Could you check a few things on this model? Use its own coordinates, in mm. A direction names the side the tool comes from. Round coordinates to 2 decimals unless told otherwise and drop trailing zeros. Loops run counter-clockwise (first coordinate to the right, second up) from the corner with the lowest first, then second, coordinate; pieces in that order, holes last. Notation, with made-up numbers: (60, 32.25) - (112, 32.25) arc R20 cw to (112, 53.25) - close; hole circle Ø4 at (-19, -15). An arc over 180 degrees is marked (long way). Use one line per item in the form item = value.
Autodesk Inventor part; units mm, degrees
ref_plane "YZ Plane" through (0, 0, 0) normal (1, 0, 0) x (0, 1, 0)
ref_plane "XZ Plane" through (0, 0, 0) normal (0, 1, 0) x (-1, 0, 0)
ref_plane "XY Plane" through (0, 0, 0) normal (0, 0, 1) x (1, 0, 0)
sketch "スケッチ1" plane through (0, 0, 0) normal (0, 0, 1) x (1, 0, 0)
  line L0 (-32.2352, 43.3932) -> (10.6011, 47.1409) construction
  line L1 (10.6011, 47.1409) -> (13.3901, 15.2627) construction
  line L2 (13.3901, 15.2627) -> (-29.4462, 11.515) construction
  line L3 (-29.4462, 11.515) -> (-32.2352, 43.3932) construction
  line L4 (-32.2352, 43.3932) -> (13.3901, 15.2627) construction
  line L5 (10.6011, 47.1409) -> (-29.4462, 11.515) construction
  line L6 (-30.8407, 27.4541) -> (11.9956, 31.2018) construction
  line L7 (7.8305, 44.389) -> (-19.0668, 42.0358) construction
  line L8 (-19.0668, 42.0358) -> (-16.7136, 15.1385) construction
  line L9 (-16.7136, 15.1385) -> (10.1837, 17.4917) construction
  line L10 (10.1837, 17.4917) -> (7.8305, 44.389) construction
  line L11 (7.8305, 44.389) -> (-16.7136, 15.1385) construction
  line L12 (-19.0668, 42.0358) -> (10.1837, 17.4917) construction
  circle A0 centre (-18.8864, 28.5) radius 10.5 construction
  circle A1 centre (-19.0668, 42.0358) radius 1.35
  line L13 (-5.6182, 43.2124) -> (-3.265, 16.3151) construction
  circle A2 centre (7.8305, 44.389) radius 1.35
  circle A3 centre (-16.7136, 15.1385) radius 1.35
  circle A4 centre (10.1837, 17.4917) radius 1.35
  arc A5 (-21.4577, 41.8266) -> (-19.0348, 39.636) centre (-19.0668, 42.0358) ccw
  arc A6 (-17.0988, 17.5074) -> (-19.0348, 39.636) centre (-18.8864, 28.5) ccw
  arc A7 (-17.0988, 17.5074) -> (-19.1136, 15.1385) centre (-16.7136, 15.1385) ccw
  line L14 (-21.4577, 41.8266) -> (-21.6756, 44.3171)
  circle A8 centre (13.1136, 8.5) radius 1.55
  circle A9 centre (13.1136, 8.5) radius 6 construction
  circle A10 centre (13.1136, 8.5) radius 4.6 construction
  line L15 (19.1136, 8.5) -> (19.1136, -8.5)
  line L16 (-19.1136, 15.1385) -> (-19.1136, -15.1385)
  line L17 (-19.1136, 0) -> (19.1136, 0) construction
  line L18 (-21.6756, 44.3171) -> (10.6011, 47.1409)
  line L19 (10.6011, 47.1409) -> (18.9683, 9.8123)
  arc A11 (19.1136, 8.5) -> (18.9683, 9.8123) centre (13.1136, 8.5) ccw
  circle A12 centre (-18.8864, -28.5) radius 10.5 construction
  circle A13 centre (-19.0668, -42.0358) radius 1.35
  circle A14 centre (7.8305, -44.389) radius 1.35
  circle A15 centre (-16.7136, -15.1385) radius 1.35
  circle A16 centre (10.1837, -17.4917) radius 1.35
  arc A17 (-19.0348, -39.636) -> (-21.4577, -41.8266) centre (-19.0668, -42.0358) ccw
  arc A18 (-19.0348, -39.636) -> (-17.0988, -17.5074) centre (-18.8864, -28.5) ccw
  arc A19 (-19.1136, -15.1385) -> (-17.0988, -17.5074) centre (-16.7136, -15.1385) ccw
  line L20 (-21.4577, -41.8266) -> (-21.6756, -44.3171)
  circle A20 centre (13.1136, -8.5) radius 1.55
  circle A21 centre (13.1136, -8.5) radius 6 construction
  line L21 (-21.6756, -44.3171) -> (10.6011, -47.1409)
  line L22 (10.6011, -47.1409) -> (18.9683, -9.8123)
  arc A22 (18.9683, -9.8123) -> (19.1136, -8.5) centre (13.1136, -8.5) ccw
  point P0 (0, 0)
  point P1 (-9.4225, 29.328)
  point P2 (-4.4416, 29.7638)
  dimension "d21" = 43
  dimension "d22" = 32
  dimension "d23" = 27
  dimension "d24" = 27
  dimension "d27" = 21
  dimension "d28" = 9.5
  dimension "d29" = 2.7
  dimension "d30" = 2.4
  dimension "d31" = 3.1
  dimension "d34" = 12
  dimension "d39" = 8.5
  dimension "d40" = 9.2
  dimension "d41" = 32
  dimension "d43" = 5
  dimension "d45" = 17
  dimension "d46" = 20
  dimension "d47" = 57
extrude "押し出し1" add sketch "スケッチ1" along normal blind 2
fillet "フィレット1" radius 2 4 edges at (-21.6756, 44.3171, 1) (-21.6756, -44.3171, 1) (10.6011, -47.1409, 1) (10.6011, 47.1409, 1)
properties part number "膝_メインフレーム_1" material "アルミニウム 2014-T4"
1. If we section it at A-A, the plane x = -10: Write out the boundary of the cut face in (y, z), plus the area to 3 significant figures.
Solution:
outline = (-45.34, 0) - (-35.21, 0) - (-35.21, 2) - (-45.34, 2) - close; (-21.79, 0) - (21.79, 0) - (21.79, 2) - (-21.79, 2) - close; (35.21, 0) - (45.34, 0) - (45.34, 2) - (35.21, 2) - close
area = 128 mm^2
2. If we section it at B-B, the plane z = 1.5: Count the separate pieces of the cut face and the enclosed holes in it, plus the area to 3 significant figures.
Solution:
separate_pieces = 1
enclosed_holes = 10
area = 2,760 mm^2
3. If we section it at D-D, the plane y = -37.5: Write out the boundary of the cut face in (x, z), plus the area to 3 significant figures.
Solution:
outline = (-12.33, 0) - (12.76, 0) - (12.76, 2) - (-12.33, 2) - close
area = 50.2 mm^2
4. We'd pull the mould along Y, two halves only. Please class faces 1 (the face through (14.545, -7.906, 0.986)), 2 (the face through (14.92, 27.87, 0.99)), 3 (the face through (19.114, 0, 1)), 4 (the face through (-5.612, -45.722, 0.986)): +Y half, -Y half, draft (parallel to the pull), parting line (faces both ways), or undercut.
Solution:
face_1 = undercut
face_2 = +Y half
face_3 = draft
face_4 = -Y half
5. If we section it at C-C, the plane y = 36: Write out the boundary of the cut face in (x, z), plus the area to 3 significant figures.
Solution:
outline = (-10.65, 0) - (13.1, 0) - (13.1, 2) - (-10.65, 2) - close
area = 47.5 mm^2
6. On a 3-axis mill with a long thin cutter (end or side, diameter ignored), from which of +Z, -Z, +X, -X, +Y, -Y can I reach the whole of each face in a straight line? I mean faces 5 (the face through (-18.557, 16.675, 0.986)), 6 (the face through (-1, 1, 2)). Say none if no direction works.
Solution:
face_5 = +Z, -Z, -X
face_6 = +Z, +X, -X, +Y, -Y
7. Please list where these lines run through material, in increasing order: line 1 along Y through (x, z) = (9.5, 1.35); line 2 along Y through (x, z) = (8, 0.8); line 3 along Y through (x, z) = (-15.5, 0.85).
Solution:
line_1 = -46.94 to -18.66, -16.33 to 16.33, 18.66 to 46.94
line_2 = -46.91 to -45.73, -43.05 to 43.05, 45.73 to 46.91
line_3 = -44.86 to -39.11, -17.89 to -15.73, -14.55 to 14.55, 15.73 to 17.89, 39.11 to 44.86
8. For P1, Ø2.5, axis at x = -16.71, y = -15.14, coming from the -Z side; P2, Ø1, axis at y = 6.5, z = 1.5, coming from the -X side, each with a flat end and sliding along its axis, tell me the tip position at first contact or that it passes through.
Solution:
P1 = through
P2 = -19.11
